from build123d import *

# Parameters (mm, degrees)
SKETCH1_R           = 1.6
BOSS_EXTRUDE1_DEPTH = 5
SKETCH5_R           = 3
CUT_EXTRUDE6_DEPTH  = 4
SKETCH2_W           = 3
SKETCH2_H           = 15
BOSS_EXTRUDE2_DEPTH = 70
SKETCH3_R           = 1.2
CUT_EXTRUDE1_DEPTH  = 70
FILLET1_R           = 10


with BuildPart() as part:
    # Sketch1 → Boss-Extrude1 (new body)
    with BuildSketch(Plane(origin=(0, 0, 0), x_dir=(1, 0, 0), z_dir=(0, 1, 0))):
        Polygon((5, 22.84134835), (16.360076307, 22.84134835), (29.991927163, 22.84134835), (29.991927163, 30.010026716), (29.991927163, 30.84134835), (24.359090043, 30.84134835), (24.359090043, 92.100281359), (24.359090043, 99.017701748), (16.360076307, 99.017701748), (16.360076307, 92.100281359), (16.360076307, 30.84134835), (-39.640909957, 30.84134835), (-39.640909957, 88.100281359), (-39.640909957, 99.017701748), (-47.640909957, 99.017701748), (-47.640909957, 88.100281359), (-47.640909957, 30.84134835), (-51.640909957, 30.84134835), (-51.640909957, 22.84134835), (-44.008072837, 22.84134835), (-35.639923693, 22.84134835), (-35.639923693, -23.088281846), (-15, -23.088281846), (-15, -30), (15, -30), (15, -23.088281846), (5, -23.088281846), align=None)
        with Locations(Location((-43.540208284, 91.841256161, 0), (0, 0, 270))):
            Circle(SKETCH1_R, mode=Mode.SUBTRACT)
        with Locations(Location((20.459791716, 91.841256161, 0), (0, 0, 270))):
            Circle(SKETCH1_R, mode=Mode.SUBTRACT)
        with Locations(Location((-43.640909957, 36.84134835, 0), (0, 0, 270))):
            Circle(SKETCH1_R, mode=Mode.SUBTRACT)
        with Locations(Location((20.359090043, 36.84134835, 0), (0, 0, 270))):
            Circle(SKETCH1_R, mode=Mode.SUBTRACT)
    extrude(amount=BOSS_EXTRUDE1_DEPTH)

    # Sketch5 → Cut-Extrude6 (cut)
    with BuildSketch(Plane.XZ):
        with Locations(Location((20.459791716, -91.841256161, 0), (0, 0, 270))):
            Circle(SKETCH5_R)
        with Locations(Location((20.359090043, -36.84134835, 0), (0, 0, 270))):
            Circle(SKETCH5_R)
        with Locations(Location((-43.540208284, -91.841256161, 0), (0, 0, 270))):
            Circle(SKETCH5_R)
        with Locations(Location((-43.640909957, -36.84134835, 0), (0, 0, 270))):
            Circle(SKETCH5_R)
    extrude(amount=-CUT_EXTRUDE6_DEPTH, mode=Mode.SUBTRACT)

    # Sketch2 → Boss-Extrude2 (add)
    with BuildSketch(Plane(origin=(0, 5, 0), x_dir=(1, 0, 0), z_dir=(0, 1, 0))):
        with Locations((0, -22.5)):
            Rectangle(SKETCH2_W, SKETCH2_H)
        with Locations((0, 22.5)):
            Rectangle(SKETCH2_W, SKETCH2_H)
    extrude(amount=BOSS_EXTRUDE2_DEPTH)

    # Sketch3 → Cut-Extrude1 (cut)
    with BuildSketch(Plane.ZY.offset(1.5)):
        with Locations((-24, 65)):
            Circle(SKETCH3_R)
        with Locations((24, 65)):
            Circle(SKETCH3_R)
    extrude(amount=-CUT_EXTRUDE1_DEPTH, mode=Mode.SUBTRACT)

    # Fillet1
    # the kernel refuses this fillet: 10 mm, written as the material it adds along each edge
    with BuildSketch(Plane(origin=(-1.5, 5, 15), x_dir=(-1, 0, 0), z_dir=(0, 0, 1)), Plane(origin=(-1.5, 5, -30), x_dir=(-1, 0, 0), z_dir=(0, 0, 1))) as fillet1_piece_1:
        with BuildLine():
            CenterArc((FILLET1_R, -FILLET1_R), FILLET1_R, 90, 90)
            Line((0, -FILLET1_R), (0, 0))
            Line((0, 0), (FILLET1_R, 0))
        make_face()
    extrude(amount=15)
    with BuildSketch(Plane(origin=(1.5, 5, 30), x_dir=(1, 0, 0), z_dir=(0, 0, -1))) as fillet1_piece_2_section:
        with BuildLine():
            CenterArc((FILLET1_R, -FILLET1_R), FILLET1_R, 90, 90)
            Line((0, -FILLET1_R), (0, 0))
            Line((0, 0), (FILLET1_R, 0))
        make_face()
    fillet1_piece_2 = extrude(amount=40, mode=Mode.PRIVATE)
    fillet1_piece_2 = split(fillet1_piece_2, bisect_by=Plane(origin=(1.5, 5, 23.088281846), z_dir=(0, 0, 1)), keep=Keep.TOP, mode=Mode.PRIVATE)
    add(fillet1_piece_2)
    with BuildSketch(Plane(origin=(1.5, 5, 30), x_dir=(1, 0, 0), z_dir=(0, 0, -1))) as fillet1_piece_3_section:
        with BuildLine():
            CenterArc((FILLET1_R, -FILLET1_R), FILLET1_R, 90, 90)
            Line((0, -FILLET1_R), (0, 0))
            Line((0, 0), (FILLET1_R, 0))
        make_face()
    fillet1_piece_3 = extrude(amount=15, mode=Mode.PRIVATE)
    fillet1_piece_3 = split(fillet1_piece_3, bisect_by=Plane(origin=(5, 5, 30), z_dir=(-1, 0, 0)), keep=Keep.TOP, mode=Mode.PRIVATE)
    add(fillet1_piece_3)
    with BuildSketch(Plane(origin=(1.5, 5, 15), x_dir=(0, 0, -1), z_dir=(-1, 0, 0)), Plane(origin=(-1.5, 5, -15), x_dir=(0, 0, 1), z_dir=(1, 0, 0))) as fillet1_piece_4:
        with BuildLine():
            CenterArc((FILLET1_R, -FILLET1_R), FILLET1_R, 90, 90)
            Line((0, -FILLET1_R), (0, 0))
            Line((0, 0), (FILLET1_R, 0))
        make_face()
    extrude(amount=3)
    with BuildSketch(Plane(origin=(1.5, 5, -15), x_dir=(1, 0, 0), z_dir=(0, 0, -1))) as fillet1_piece_5_section:
        with BuildLine():
            CenterArc((FILLET1_R, -FILLET1_R), FILLET1_R, 90, 90)
            Line((0, -FILLET1_R), (0, 0))
            Line((0, 0), (FILLET1_R, 0))
        make_face()
    fillet1_piece_5 = extrude(amount=15, mode=Mode.PRIVATE)
    fillet1_piece_5 = split(fillet1_piece_5, bisect_by=Plane(origin=(5, 5, -15), z_dir=(-1, 0, 0)), keep=Keep.TOP, mode=Mode.PRIVATE)
    add(fillet1_piece_5)
    with BuildSketch(Plane(origin=(1.5, 5, 10), x_dir=(1, 0, 0), z_dir=(0, 0, -1))) as fillet1_piece_6_section:
        with BuildLine():
            CenterArc((FILLET1_R, -FILLET1_R), FILLET1_R, 90, 90)
            Line((0, -FILLET1_R), (0, 0))
            Line((0, 0), (FILLET1_R, 0))
        make_face()
    fillet1_piece_6 = extrude(amount=40, mode=Mode.PRIVATE)
    fillet1_piece_6 = split(fillet1_piece_6, bisect_by=Plane(origin=(1.5, 5, -22.84134835), z_dir=(0, 0, -1)), keep=Keep.TOP, mode=Mode.PRIVATE)
    add(fillet1_piece_6)
    with BuildSketch(Plane(origin=(1.5, 5, 15), x_dir=(0, 0, -1), z_dir=(-1, 0, 0))) as fillet1_piece_7a_section:
        with BuildLine():
            CenterArc((FILLET1_R, -FILLET1_R), FILLET1_R, 90, 90)
            Line((0, -FILLET1_R), (0, 0))
            Line((0, 0), (FILLET1_R, 0))
        make_face()
    fillet1_piece_7a = extrude(amount=28, mode=Mode.PRIVATE)
    fillet1_piece_7a = split(fillet1_piece_7a, bisect_by=Plane(origin=(-1.5, 5, 15), z_dir=(-1, 0, 0)), keep=Keep.TOP, mode=Mode.PRIVATE)
    with BuildSketch(Plane(origin=(-1.5, 5, -10), x_dir=(-1, 0, 0), z_dir=(0, 0, 1))) as fillet1_piece_7b_section:
        with BuildLine():
            CenterArc((FILLET1_R, -FILLET1_R), FILLET1_R, 90, 90)
            Line((0, -FILLET1_R), (0, 0))
            Line((0, 0), (FILLET1_R, 0))
        make_face()
    fillet1_piece_7b = extrude(amount=40, mode=Mode.PRIVATE)
    fillet1_piece_7b = split(fillet1_piece_7b, bisect_by=Plane(origin=(-1.5, 5, 15), z_dir=(0, 0, -1)), keep=Keep.TOP, mode=Mode.PRIVATE)
    fillet1_piece_7 = fillet1_piece_7a & fillet1_piece_7b
    add(fillet1_piece_7)
    with BuildSketch(Plane(origin=(1.5, 5, 30), x_dir=(1, 0, 0), z_dir=(0, 0, -1))) as fillet1_piece_8a_section:
        with BuildLine():
            CenterArc((FILLET1_R, -FILLET1_R), FILLET1_R, 90, 90)
            Line((0, -FILLET1_R), (0, 0))
            Line((0, 0), (FILLET1_R, 0))
        make_face()
    fillet1_piece_8a = extrude(amount=40, mode=Mode.PRIVATE)
    fillet1_piece_8a = split(fillet1_piece_8a, bisect_by=Plane(origin=(5, 5, 30), z_dir=(-1, 0, 0)), keep=Keep.TOP, mode=Mode.PRIVATE)
    fillet1_piece_8a = split(fillet1_piece_8a, bisect_by=Plane(origin=(1.5, 5, 15), z_dir=(0, 0, -1)), keep=Keep.TOP, mode=Mode.PRIVATE)
    with BuildSketch(Plane(origin=(26.5, 5, 15), x_dir=(0, 0, -1), z_dir=(-1, 0, 0))) as fillet1_piece_8b_section:
        with BuildLine():
            CenterArc((FILLET1_R, -FILLET1_R), FILLET1_R, 90, 90)
            Line((0, -FILLET1_R), (0, 0))
            Line((0, 0), (FILLET1_R, 0))
        make_face()
    fillet1_piece_8b = extrude(amount=28, mode=Mode.PRIVATE)
    fillet1_piece_8b = split(fillet1_piece_8b, bisect_by=Plane(origin=(5, 5, 15), z_dir=(-1, 0, 0)), keep=Keep.TOP, mode=Mode.PRIVATE)
    fillet1_piece_8b = split(fillet1_piece_8b, bisect_by=Plane(origin=(1.5, 5, 15), z_dir=(1, 0, 0)), keep=Keep.TOP, mode=Mode.PRIVATE)
    fillet1_piece_8 = fillet1_piece_8a & fillet1_piece_8b
    add(fillet1_piece_8)
    with BuildSketch(Plane(origin=(-26.5, 5, -15), x_dir=(0, 0, 1), z_dir=(1, 0, 0))) as fillet1_piece_9a_section:
        with BuildLine():
            CenterArc((FILLET1_R, -FILLET1_R), FILLET1_R, 90, 90)
            Line((0, -FILLET1_R), (0, 0))
            Line((0, 0), (FILLET1_R, 0))
        make_face()
    fillet1_piece_9a = extrude(amount=28, mode=Mode.PRIVATE)
    fillet1_piece_9a = split(fillet1_piece_9a, bisect_by=Plane(origin=(-1.5, 5, -15), z_dir=(-1, 0, 0)), keep=Keep.TOP, mode=Mode.PRIVATE)
    with BuildSketch(Plane(origin=(-1.5, 5, -30), x_dir=(-1, 0, 0), z_dir=(0, 0, 1))) as fillet1_piece_9b_section:
        with BuildLine():
            CenterArc((FILLET1_R, -FILLET1_R), FILLET1_R, 90, 90)
            Line((0, -FILLET1_R), (0, 0))
            Line((0, 0), (FILLET1_R, 0))
        make_face()
    fillet1_piece_9b = extrude(amount=40, mode=Mode.PRIVATE)
    fillet1_piece_9b = split(fillet1_piece_9b, bisect_by=Plane(origin=(-1.5, 5, -15), z_dir=(0, 0, 1)), keep=Keep.TOP, mode=Mode.PRIVATE)
    fillet1_piece_9 = fillet1_piece_9a & fillet1_piece_9b
    add(fillet1_piece_9)
    with BuildSketch(Plane(origin=(-1.5, 5, -15), x_dir=(0, 0, 1), z_dir=(1, 0, 0))) as fillet1_piece_10a_section:
        with BuildLine():
            CenterArc((FILLET1_R, -FILLET1_R), FILLET1_R, 90, 90)
            Line((0, -FILLET1_R), (0, 0))
            Line((0, 0), (FILLET1_R, 0))
        make_face()
    fillet1_piece_10a = extrude(amount=28, mode=Mode.PRIVATE)
    fillet1_piece_10a = split(fillet1_piece_10a, bisect_by=Plane(origin=(5, 5, -15), z_dir=(-1, 0, 0)), keep=Keep.TOP, mode=Mode.PRIVATE)
    fillet1_piece_10a = split(fillet1_piece_10a, bisect_by=Plane(origin=(1.5, 5, -15), z_dir=(1, 0, 0)), keep=Keep.TOP, mode=Mode.PRIVATE)
    with BuildSketch(Plane(origin=(1.5, 5, 10), x_dir=(1, 0, 0), z_dir=(0, 0, -1))) as fillet1_piece_10b_section:
        with BuildLine():
            CenterArc((FILLET1_R, -FILLET1_R), FILLET1_R, 90, 90)
            Line((0, -FILLET1_R), (0, 0))
            Line((0, 0), (FILLET1_R, 0))
        make_face()
    fillet1_piece_10b = extrude(amount=40, mode=Mode.PRIVATE)
    fillet1_piece_10b = split(fillet1_piece_10b, bisect_by=Plane(origin=(5, 5, 10), z_dir=(-1, 0, 0)), keep=Keep.TOP, mode=Mode.PRIVATE)
    fillet1_piece_10b = split(fillet1_piece_10b, bisect_by=Plane(origin=(1.5, 5, -15), z_dir=(0, 0, 1)), keep=Keep.TOP, mode=Mode.PRIVATE)
    fillet1_piece_10 = fillet1_piece_10a & fillet1_piece_10b
    add(fillet1_piece_10)


solid = part.part
Work out the finished part from the listing and answer in its coordinate system (mm). A direction names the side the tool comes from. Coordinates: 2 decimals unless noted, no trailing zeros. Write each loop counter-clockwise with the first axis right and the second up, starting at its lowest first coordinate (ties: lowest second). Pieces come first, ordered by that corner, then holes. Notation, with made-up numbers: M 5.25,-39.75 L 63.25,-39.75 A23 cw 63.25,-17.75 Z; hole C 16.25,-19 d1. An arc over 180 degrees is marked long. Answer as CSV lines item,"result". Start each with the question number.
Item 1: Section C-C on z = -18 is taken. Write down the section's boundary in (x, y), and give its area (3 significant figures).
Item 2: Flat-ended cylindrical pins translate along their axes: P1, Ø1.8, axis at x = -42.5, z = -35.5, coming from the -Y side; P2, Ø6, axis at x = -27, z = -35.5, coming from the -Y side; P3, Ø3, axis at y = 58, z = -14, coming from the +X side; P4, Ø2, axis at x = 22, y = 5, coming from the +Z side. Find the tip coordinate at first contact, or state that the pin passes through.
Item 3: Section B-B on z = -51 is taken. Write down the section's boundary in (x, y), and give its area (3 significant figures).
Item 4: A tool of negligible diameter and unlimited length cuts with its end or side. For faces 4 (the face through (-1.5, 45, -22)), 5 (the face through (-44, 2, -22.841)), 6 (the face through (-44.689, 1.972, -94.612)), 7 (the face through (0, 45, 15)), from which of +Z, -Z, +X, -X, +Y, -Y can it reach the whole face along a straight path? Write none if from no direction.
Item 5: Consider L1, parallel to Z at x = -0.65, y = 65; L2, parallel to Y at x = 0.4, z = -24; L3, parallel to Y at x = -32.5, z = -3.5. Determine where each line is inside the solid, lowest interval first.
Item 6: Section A-A on y = 16.5 is taken. Write down the section's boundary in (x, z).
Item 7: Determine the mould class of faces 1 (the face through (-1.5, 45, 23)), 2 (the face through (20.491, 1.972, -33.844)), 3 (the face through (24.359, 2, -64)) for opening direction X: released by +X, released by -X, zero draft, split by the parting line, or undercut.
Checks:
1,outline,"M -35.64,0 L 5,0 L 5,7.4 A10 cw 1.5,15 L 1.5,75 L -1.5,75 L -1.5,15 A10 cw -11.5,5 L -35.64,5 Z"
1,area,"451 mm²"
2,P1,"stops at y = 4"
2,P2,"passes through"
2,P3,"stops at x = 1.5"
2,P4,"stops at z = -22.84"
3,outline,"M -47.64,0 L -39.64,0 L -39.64,5 L -47.64,5 Z; M 16.36,0 L 24.36,0 L 24.36,5 L 16.36,5 Z"
3,area,"80.0 mm²"
4,face 4,"+Z, -Z, -X, +Y"
4,face 5,"+Z, -X, +Y, -Y"
4,face 6,"-Y"
4,face 7,"+X, -X, +Y"
5,L1,"z = -30 to -25.2, -22.8 to -15, 15 to 22.8, 25.2 to 30"
5,L2,"y = 0 to 63.8, 66.2 to 75"
5,L3,"y = 0 to 5"
6,outline,"M -1.5,-30 L 1.5,-30 L 1.5,-15 L -1.5,-15 Z; M -1.5,15 L 1.5,15 L 1.5,30 L -1.5,30 Z"
7,face 1,"released by -X"
7,face 2,"undercut"
7,face 3,"released by +X"
